from build123d import *

# Parameters (mm, degrees)
SKETCH1_W           = 17
SKETCH1_H           = 65
SKETCH1_R           = 2.1
SKETCH1_W_2         = 60
SKETCH1_H_2         = 15
SKETCH1_H_3         = 6
BOSS_EXTRUDE1_DEPTH = 3
SKETCH2_W           = 17
SKETCH2_H           = 65
SKETCH2_R           = 2.1
BOSS_EXTRUDE2_DEPTH = 3.8
SKETCH3_R           = 2.1
CUT_EXTRUDE1_DEPTH  = 18.8
CUT_EXTRUDE2_DEPTH  = 3
SKETCH5_W           = 1
SKETCH5_H           = 1
SKETCH5_W_2         = 15
SKETCH5_H_2         = 64
SKETCH5_H_3         = 14
SKETCH5_W_3         = 58
CUT_EXTRUDE3_DEPTH  = 3.8


with BuildPart() as part:
    # Sketch1 → Boss-Extrude1 (new body)
    with BuildSketch(Plane(origin=(0, 0, 0), x_dir=(1, 0, 0), z_dir=(0, 1, 0))):
        Polygon((-8.5, 72.5), (-30, 7.5), (-8.5, 7.5), align=None)
        Polygon((8.5, 7.5), (30, 7.5), (8.5, 72.5), align=None)
        with Locations((0, 40)):
            Rectangle(SKETCH1_W, SKETCH1_H)
        with Locations((0, 22.5)):
            Circle(SKETCH1_R, mode=Mode.SUBTRACT)
        with Locations((0, 57.5)):
            Circle(SKETCH1_R, mode=Mode.SUBTRACT)
        Rectangle(SKETCH1_W_2, SKETCH1_H_2)
        with Locations((-20, 0)):
            Circle(SKETCH1_R, mode=Mode.SUBTRACT)
        with Locations((20, 0)):
            Circle(SKETCH1_R, mode=Mode.SUBTRACT)
        with Locations((0, -10.5)):
            Rectangle(SKETCH1_W_2, SKETCH1_H_3)
        with Locations((0, 57.5)):
            Circle(SKETCH1_R)
        with Locations((0, 22.5)):
            Circle(SKETCH1_R)
        with Locations((-20, 0)):
            Circle(SKETCH1_R)
        with Locations((20, 0)):
            Circle(SKETCH1_R)
    extrude(amount=BOSS_EXTRUDE1_DEPTH)

    # Sketch2 → Boss-Extrude2 (add)
    with BuildSketch(Plane(origin=(0, 3, 0), x_dir=(1, 0, 0), z_dir=(0, 1, 0))):
        with Locations((0, 40)):
            Rectangle(SKETCH2_W, SKETCH2_H)
        with Locations((0, 22.5)):
            Circle(SKETCH2_R, mode=Mode.SUBTRACT)
        with Locations((0, 57.5)):
            Circle(SKETCH2_R, mode=Mode.SUBTRACT)
        Polygon((-8.5, 7.5), (-30, 7.5), (-30, -7.5), (30, -7.5), (30, 7.5), (8.5, 7.5), align=None)
        with Locations((-20, 0)):
            Circle(SKETCH2_R, mode=Mode.SUBTRACT)
        with Locations((20, 0)):
            Circle(SKETCH2_R, mode=Mode.SUBTRACT)
    extrude(amount=BOSS_EXTRUDE2_DEPTH)

    # Sketch3 → Cut-Extrude1 (cut)
    with BuildSketch(Plane(origin=(0, 6.8, 0), x_dir=(1, 0, 0), z_dir=(0, 1, 0))):
        with Locations((0, 57.5)):
            Circle(SKETCH3_R)
        with Locations((0, 22.5)):
            Circle(SKETCH3_R)
        with Locations((20, 0)):
            Circle(SKETCH3_R)
        with Locations((-20, 0)):
            Circle(SKETCH3_R)
    extrude(amount=-CUT_EXTRUDE1_DEPTH, mode=Mode.SUBTRACT)

    # Sketch4 → Cut-Extrude2 (cut)
    with BuildSketch(Plane(origin=(0, 0, 0), x_dir=(-1, 0, 0), z_dir=(0, -1, 0))):
        Polygon((23.6, 2.1), (23.6, -2.1), (20, -4.1), (16.4, -2.1), (16.4, 2.1), (20, 4.1), align=None)
        Polygon((-23.6, 2.1), (-23.6, -2.1), (-20, -4.1), (-16.4, -2.1), (-16.4, 2.1), (-20, 4.1), align=None)
        Polygon((0, 18.4), (3.6, 20.4), (3.6, 24.6), (0, 26.6), (-3.6, 24.6), (-3.6, 20.4), align=None)
        Polygon((3.6, 55.4), (3.6, 59.6), (0, 61.6), (-3.6, 59.6), (-3.6, 55.4), (0, 53.4), align=None)
    extrude(amount=-CUT_EXTRUDE2_DEPTH, mode=Mode.SUBTRACT)

    # Sketch5 → Cut-Extrude3 (cut)
    with BuildSketch(Plane(origin=(0, 6.8, 0), x_dir=(1, 0, 0), z_dir=(0, 1, 0))):
        with Locations((8, 72)):
            Rectangle(SKETCH5_W, SKETCH5_H)
        with Locations((0, 72)):
            Rectangle(SKETCH5_W_2, SKETCH5_H)
        with Locations((-8, 72)):
            Rectangle(SKETCH5_W, SKETCH5_H)
        with Locations((-8, 39.5)):
            Rectangle(SKETCH5_W, SKETCH5_H_2)
        with Locations((8, 39.5)):
            Rectangle(SKETCH5_W, SKETCH5_H_2)
        with Locations((29.5, -7)):
            Rectangle(SKETCH5_W, SKETCH5_H)
        with Locations((-29.5, -7)):
            Rectangle(SKETCH5_W, SKETCH5_H)
        with Locations((-29.5, 0.5)):
            Rectangle(SKETCH5_W, SKETCH5_H_3)
        with Locations((0, -7)):
            Rectangle(SKETCH5_W_3, SKETCH5_H)
        with Locations((29.5, 0.5)):
            Rectangle(SKETCH5_W, SKETCH5_H_3)
    extrude(amount=-CUT_EXTRUDE3_DEPTH, mode=Mode.SUBTRACT)


solid = part.part
The model under review builds one solid part; all positions refer to its coordinate system, in mm. A direction names the side the tool comes from. Round coordinates to 2 decimals unless told otherwise and drop trailing zeros. Loops run counter-clockwise (first coordinate to the right, second up) from the corner with the lowest first, then second, coordinate; pieces in that order, holes last. Notation, with made-up numbers: (-29.5, 51.25) -> (15.5, 51.25) arc R7 cw to (15.5, 63.25) -> close; hole circle Ø9 at (70, -40). An arc over 180 degrees is marked (long way). Write item = value, one per line. Start each with the question number.
Item 1: To check wall thickness, follow L1, parallel to X at y = 3.25, z = 0; L2, parallel to Z at x = 0, y = 5.35; L3, parallel to X at y = 6, z = -22.5. State the ranges of each line that lie inside material, in increasing order.
Item 2: Insertion check: pin 1 (1.9 mm diameter, centred on y = 4.5, z = -39, fed in from -X); pin 2 (2.5 mm diameter, centred on y = 2, z = -23, fed in from -X); pin 3 (1 mm diameter, centred on x = 11, z = -36, fed in from +Y). Each pin has a flat end and moves straight along its axis. Give the tip position at first contact, or say it passes through.
Item 3: Take a section at C-C on x = -5. Give the boundary of the cut face in (y, z).
Item 4: Mouldability with a two-part tool opening along Z and no side actions: class faces 4 (the flat face through (-7.5, 5, -39)), 5 (the flat face through (0, 5, 6.5)), 6 (the flat face through (1.8, 1.5, -19.4)) as released by +Z, released by -Z, zero draft, split by the parting line, or undercut.
Item 5: Take a section at D-D on z = -66. Give the boundary of the cut face in (x, y).
Item 6: For faces 1 (the cylindrical face through (-0.46, 4.87, -55.45)), 2 (the flat face through (-18, 5, -7.5)), 3 (the flat face through (-2, 3, -21)), list the 3-axis set-ups (+Z, -Z, +X, -X, +Y, -Y) from which the entire face can be reached by the end or side of a thin tool; tool diameter is ignored.
Item 7: Take a section at B-B on y = 1.75. Count the separate pieces of the cut face and the enclosed holes in it, plus the area to 3 significant figures.
Item 8: Take a section at A-A on z = 0. Give the boundary of the cut face in (x, y), plus the area to 3 significant figures.
Result:
q1.L1 = -29 to -22.1, -17.9 to 17.9, 22.1 to 29
q1.L2 = -71.5 to -59.6, -55.4 to -24.6, -20.4 to 6.5
q1.L3 = -7.5 to -2.1, 2.1 to 7.5
q2.pin_1 = -7.5
q2.pin_2 = -25.29
q2.pin_3 = 3
q3.outline = (0, -72.5) -> (3, -72.5) -> (3, -71.5) -> (6.8, -71.5) -> (6.8, 6.5) -> (3, 6.5) -> (3, 13.5) -> (0, 13.5) -> close
q4.face_4 = zero draft
q4.face_5 = released by +Z
q4.face_6 = undercut
q5.outline = (-10.65, 0) -> (10.65, 0) -> (10.65, 3) -> (7.5, 3) -> (7.5, 6.8) -> (-7.5, 6.8) -> (-7.5, 3) -> (-10.65, 3) -> close
q6.face_1 = +Y, -Y
q6.face_2 = -Z, -X, +Y
q6.face_3 = -Y
q7.separate_pieces = 1
q7.enclosed_holes = 4
q7.area = 3,580 mm²
q8.outline = (-30, 0) -> (-23.6, 0) -> (-23.6, 3) -> (-22.1, 3) -> (-22.1, 6.8) -> (-29, 6.8) -> (-29, 3) -> (-30, 3) -> close; (-17.9, 3) -> (-16.4, 3) -> (-16.4, 0) -> (16.4, 0) -> (16.4, 3) -> (17.9, 3) -> (17.9, 6.8) -> (-17.9, 6.8) -> close; (22.1, 3) -> (23.6, 3) -> (23.6, 0) -> (30, 0) -> (30, 3) -> (29, 3) -> (29, 6.8) -> (22.1, 6.8) -> close
q8.area = 325 mm²
